Check sheet for the modelled part. Datum: model origin and axes. Units: mm. Give positions to 0.01 mm unless a question says otherwise; leave off trailing zeros. Loops run counter-clockwise (first coordinate to the right, second up) from the corner with the lowest first, then second, coordinate; pieces in that order, holes last. Notation, with made-up numbers: (10.5, -28) - (64.5, -28) arc R7 ccw to (64.5, -20) - close; hole circle Ø10 at (20, -7.75). An arc over 180 degrees is marked (long way). Answer in a Markdown table with one row per item. Add a question column.
(1) Go/stop test with flat-tipped pins: P1, Ø1.9, axis at x = 195.5, y = 3, coming from the -Z side; P2, Ø1.9, axis at y = 4.5, z = -245.5, coming from the +X side; P3, Ø3, axis at y = 5, z = -244.5, coming from the -X side. Record where each tip stops, or that it passes through.
(2) Sectioned sample at B-B on y = 2.25. State how many separate pieces and enclosed holes the cut face has, then the cut area to 3 significant figures.
(3) Sectioned sample at A-A on z = 117.5. Enter the section's corners in (x, y).
(4) Thickness scan on L1, parallel to X at y = 3.75, z = 124.5; L2, parallel to Z at x = 139.5, y = 4.75; L3, parallel to X at y = 3, z = 175. Record the ranges inside material, lowest first.
from build123d import *

# Parameters (mm, degrees)
SKETCH2_W                         = 400
SKETCH2_H                         = 500
BOSS_EXTRUDE2_DEPTH               = 6.35
M3_5X0_6_TAPPED_HOLE2_D           = 2.9
M3_5X0_6_TAPPED_HOLE2_CSINK_D     = 3.55
M3_5X0_6_TAPPED_HOLE2_CSINK_ANGLE = 90
CHAMFER1_SIZE                     = 25
SKETCH9_W                         = 6.35
SKETCH9_H                         = 36
SKETCH9_W_2                       = 36
SKETCH9_H_2                       = 6.35
CUT_EXTRUDE1_DEPTH                = 321.219178845


with BuildPart() as part:
    # Sketch2 → Boss-Extrude2 (new body)
    with BuildSketch(Plane(origin=(0, 0, 0), x_dir=(1, 0, 0), z_dir=(0, 1, 0))):
        Rectangle(SKETCH2_W, SKETCH2_H)
    extrude(amount=BOSS_EXTRUDE2_DEPTH)

    # M3.5x0.6 Tapped Hole2 (through all)
    with Locations(Plane(origin=(0, 6.35, 0), x_dir=(1, 0, 0), z_dir=(0, 1, 0))):
        with Locations((-139.5, 175), (139.5, 175), (-139.5, -175), (139.5, -175)):
            CounterSinkHole(M3_5X0_6_TAPPED_HOLE2_D / 2, M3_5X0_6_TAPPED_HOLE2_CSINK_D / 2, counter_sink_angle=M3_5X0_6_TAPPED_HOLE2_CSINK_ANGLE)

    # Chamfer1
    chamfer1_edges = [part.edges().sort_by_distance(p)[0] for p in [
        (200, 3.175, 250),
        (-200, 3.175, 250),
        (-200, 3.175, -250),
        (200, 3.175, -250),
    ]]
    chamfer(chamfer1_edges, length=CHAMFER1_SIZE)

    # Sketch9 → Cut-Extrude1 (cut, through all)
    with BuildSketch(Plane(origin=(0, 6.35, 0), x_dir=(1, 0, 0), z_dir=(0, 1, 0))):
        with Locations((194.825, 117)):
            Rectangle(SKETCH9_W, SKETCH9_H)
        with Locations((102, -244.825)):
            Rectangle(SKETCH9_W_2, SKETCH9_H_2)
        with Locations((-102, -244.825)):
            Rectangle(SKETCH9_W_2, SKETCH9_H_2)
        with Locations((-102, 244.825)):
            Rectangle(SKETCH9_W_2, SKETCH9_H_2)
        with Locations((102, 244.825)):
            Rectangle(SKETCH9_W_2, SKETCH9_H_2)
        with Locations((194.825, -117)):
            Rectangle(SKETCH9_W, SKETCH9_H)
        with Locations((-194.825, -117)):
            Rectangle(SKETCH9_W, SKETCH9_H)
        with Locations((-194.825, 117)):
            Rectangle(SKETCH9_W, SKETCH9_H)
    extrude(amount=-CUT_EXTRUDE1_DEPTH, mode=Mode.SUBTRACT)


solid = part.part
Reply:
| question | item | result |
|---|---|---|
| 1 | P1 | z = -230.45 |
| 1 | P2 | x = 180.45 |
| 1 | P3 | x = -182 |
| 2 | separate pieces | 1 |
| 2 | enclosed holes | 12 |
| 2 | area | 197,000 mm^2 |
| 3 | outline | (-200, 0) - (-198, 0) - (-198, 6.35) - (-200, 6.35) - close; (-191.65, 0) - (191.65, 0) - (191.65, 6.35) - (-191.65, 6.35) - close; (198, 0) - (200, 0) - (200, 6.35) - (198, 6.35) - close |
| 4 | L1 | -200 to -198, -191.65 to 191.65, 198 to 200 |
| 4 | L2 | -250 to -176.45, -173.55 to 173.55, 176.45 to 250 |
| 4 | L3 | -200 to -140.95, -138.05 to 138.05, 140.95 to 200 |
